```python
from build123d import *

# Parameters (mm, degrees)
F0_R     = 53
F0_R_2   = 51.5
F1_DEPTH = 15
F3_R     = 3.5
F4_DEPTH = 7
F5_R     = 1


with BuildPart() as f1:
    # F0 (on Top) → F1 (new body)
    with BuildSketch(Plane.XY):
        Circle(F0_R)
        Circle(F0_R_2, mode=Mode.SUBTRACT)
    extrude(amount=F1_DEPTH)

    # F3 (on offset) → F4 (join)
    with BuildSketch(Plane.YZ.offset(51.5)):
        with Locations((0, 7.729115)):
            Circle(F3_R)
    extrude(amount=F4_DEPTH)

    # F5
    f5_edges = [f1.edges().sort_by_distance(p)[0] for p in [
        (58.5, -3.5, 7.729115),
    ]]
    fillet(f5_edges, radius=F5_R)


solid = f1.part
```
Source: CAD feature listing. Evaluate the final solid. Frame: model axes, mm. A direction names the side the tool comes from. Coordinates: 2 decimals unless noted, no trailing zeros. Order: outer loops, then holes, each group sorted by start corner. A loop starts at its lowest first (then second) coordinate and runs counter-clockwise, first axis right, second up. Notation, with made-up numbers: (47, 42.25) - (103, 42.25) arc R28 ccw to (103, 77.25) - close; hole circle Ø4 at (-5.75, 19). An arc over 180 degrees is marked (long way). One line per item, written item: value.
1) Mould query, pull axis X, two halves, no side actions, for faces 3 (the face through (-8.1, 51.3, 15)), 4 (the face through (28, 45, 7)), 5 (the face through (-11.164, -50.275, 7.395)), 6 (the face through (58.5, 0, 8)). Classes: released by +X, released by -X, zero draft, split by the parting line, or undercut.
Computed values:
face 3: zero draft
face 4: split by the parting line
face 5: undercut
face 6: released by +X
2) Cut plane B-B on x = 0. Output: boundary loops of the cut face in (y, z), plus the area to 3 significant figures.
Computed values:
outline: (-53, 0) - (-51.5, 0) - (-51.5, 15) - (-53, 15) - close; (51.5, 0) - (53, 0) - (53, 15) - (51.5, 15) - close
area: 45.0 mm^2
3) Ray query, line 1 (X direction, y = -1.5, z = 7.5); line 2 (X direction, y = 1, z = 11.25); line 3 (Y direction, x = 0, z = 3.75). Return the intervals inside material, ascending. Write a range as [from, to].
Computed values:
line 1: x = [-52.98, -51.48], [51.48, 58.5]
line 2: x = [-52.99, -51.49], [51.49, 52.99]
line 3: y = [-53, -51.5], [51.5, 53]
4) Contact query for flat-ended pins moving along their axis: pin 1 (1.5 mm diameter, centred on y = -11, z = 7.5, fed in from -X); pin 2 (5 mm diameter, centred on x = 38, z = 6, fed in from -Y); pin 3 (6 mm diameter, centred on y = -26, z = 5, fed in from +X). Output: stop coordinate, or through.
Computed values:
pin 1: stops at x = -52
pin 2: stops at y = -39.35
pin 3: stops at x = 47.75
5) Cut plane C-C on y = 25.5. Output: boundary loops of the cut face in (x, z), plus the area to 3 significant figures.
Computed values:
outline: (-46.46, 0) - (-44.74, 0) - (-44.74, 15) - (-46.46, 15) - close; (44.74, 0) - (46.46, 0) - (46.46, 15) - (44.74, 15) - close
area: 51.6 mm^2
6) Cut plane A-A on y = 0. Output: boundary loops of the cut face in (x, z).
Computed values:
outline: (-53, 0) - (-51.5, 0) - (-51.5, 15) - (-53, 15) - close; (51.5, 0) - (53, 0) - (53, 4.23) - (57.5, 4.23) arc R1 ccw to (58.5, 5.23) - (58.5, 10.23) arc R1 ccw to (57.5, 11.23) - (53, 11.23) - (53, 15) - (51.5, 15) - close
7) Reachability of faces 1 (the face through (55.16, -0.759, 4.312)), 2 (the face through (-8.1, 51.3, 0)) from +Z, -Z, +X, -X, +Y, -Y: full face, straight path, thin tool, end or side. Return the list, or none.
Computed values:
face 1: +X
face 2: -Z, +X, -X, +Y, -Y
